Build history of the part. All positions in model axes, mm. A direction names the side the tool comes from. Give positions to 0.01 mm unless a question says otherwise; leave off trailing zeros. Write each loop counter-clockwise with the first axis right and the second up, starting at its lowest first coordinate (ties: lowest second). Pieces come first, ordered by that corner, then holes. Notation, with made-up numbers: (28, 81) - (81, 81) arc R17 ccw to (81, 98) - close; hole circle Ø10 at (62.5, 21). An arc over 180 degrees is marked (long way). Use one line per item in the form item = value. Start each with the question number.
from build123d import *

# Parameters (mm, degrees)
SKETCH5_W           = 31.8
SKETCH5_H           = 12.7
BOSS_EXTRUDE4_DEPTH = 31.8
SKETCH6_R           = 3.175
BOSS_EXTRUDE5_DEPTH = 9.8
SKETCH10_R          = 3.175
BOSS_EXTRUDE6_DEPTH = 9.8


with BuildPart() as part:
    # Sketch5 → Boss-Extrude4 (new body)
    with BuildSketch(Plane.XY):
        with Locations((-44.843150914, -10.871383787)):
            Rectangle(SKETCH5_W, SKETCH5_H)
    extrude(amount=BOSS_EXTRUDE4_DEPTH)

    # Sketch6 → Boss-Extrude5 (add)
    with BuildSketch(Plane.XY.offset(31.8)):
        with Locations((-44.843150914, -10.871383787)):
            Circle(SKETCH6_R)
    boss_extrude5 = extrude(amount=BOSS_EXTRUDE5_DEPTH)

    # Mirror1: Boss-Extrude5 across plane
    add(boss_extrude5.mirror(Plane.XY.offset(15.9)))

    # Sketch10 → Boss-Extrude6 (add)
    with BuildSketch(Plane(origin=(-28.943150914, 0, 0), x_dir=(0, 0, -1), z_dir=(1, 0, 0))):
        with Locations((-15.9, -10.871383787)):
            Circle(SKETCH10_R)
    boss_extrude6 = extrude(amount=BOSS_EXTRUDE6_DEPTH)

    # Mirror2: Boss-Extrude6 across plane
    add(boss_extrude6.mirror(Plane(origin=(-44.843150914, 0, 0), x_dir=(0, 0, 1), z_dir=(1, 0, 0))))


solid = part.part
(1) Cut at C-C, the plane y = -15.5. Give the cut face in (x, z), then the cut area to 3 significant figures.
(2) Cut at A-A, the plane z = 15.9. Give the cut face in (x, y), then the cut area to 3 significant figures.
(3) Pin check, flat tips, straight feed: pin 1 Ø1 at (y, z) = (-6.5, 7.5) entering from -X; pin 2 Ø2 at (x, y) = (-64, -12) entering from -Z; pin 3 Ø2 at (y, z) = (-6.5, 16) entering from +X; pin 4 Ø5 at (x, z) = (-56, -4) entering from +Y. Stop position of each tip, or through.
(4) Which spindle directions (+Z, -Z, +X, -X, +Y, -Y) get a long thin tool onto all of the face, cutting with end or side? Do faces 1 (the cylindrical face through (-47.183, -8.726, -4.831)), 2 (the cylindrical face through (-65.575, -8.726, 18.24)), 3 (the cylindrical face through (-47.183, -8.726, 36.631)). Say none if no direction does.
(5) Wall check: line 1 (X direction, y = -12.5, z = 2); line 2 (Z direction, x = -52, y = -5.5); line 3 (X direction, y = -8.75, z = 32.5). Give the ranges that are in metal, low to high. Write a range as from..to.
(6) Cut at B-B, the plane x = -46. Give the cut face in (y, z).
(7) Cut at D-D, the plane z = 4. Give the cut face in (x, y), then the cut area to 3 significant figures.
Solution:
q1.outline = (-60.74, 0) - (-28.94, 0) - (-28.94, 31.8) - (-60.74, 31.8) - close
q1.area = 1,010 mm2
q2.outline = (-70.54, -14.05) - (-60.74, -14.05) - (-60.74, -17.22) - (-28.94, -17.22) - (-28.94, -14.05) - (-19.14, -14.05) - (-19.14, -7.7) - (-28.94, -7.7) - (-28.94, -4.52) - (-60.74, -4.52) - (-60.74, -7.7) - (-70.54, -7.7) - close
q2.area = 528 mm2
q3.pin_1 = -60.74
q3.pin_2 = 12.73
q3.pin_3 = -28.94
q3.pin_4 = through
q4.face_1 = -Z
q4.face_2 = -X
q4.face_3 = +Z
q5.line_1 = -60.74..-28.94
q5.line_2 = 0..31.8
q5.line_3 = -47.21..-42.48
q6.outline = (-17.22, 0) - (-13.83, 0) - (-13.83, -9.8) - (-7.91, -9.8) - (-7.91, 0) - (-4.52, 0) - (-4.52, 31.8) - (-7.91, 31.8) - (-7.91, 41.6) - (-13.83, 41.6) - (-13.83, 31.8) - (-17.22, 31.8) - close
q7.outline = (-60.74, -17.22) - (-28.94, -17.22) - (-28.94, -4.52) - (-60.74, -4.52) - close
q7.area = 404 mm2
